Part model, mm, in its own coordinate system. A direction names the side the tool comes from. Round coordinates to 2 decimals unless told otherwise and drop trailing zeros. Loops run counter-clockwise (first coordinate to the right, second up) from the corner with the lowest first, then second, coordinate; pieces in that order, holes last. Notation, with made-up numbers: (13.25, 31.25) -> (19.25, 31.25) arc R18 cw to (19.25, 60.25) -> close; hole circle Ø5 at (8, 1.25). An arc over 180 degrees is marked (long way). Use a Markdown table: item, result. Add a question column.
Item 1: Flat gauge pins, fed straight in: pin 1 (6 mm diameter, centred on y = -8.5, z = -14.5, fed in from +X); pin 2 (5 mm diameter, centred on x = 40.5, y = 12, fed in from -Z); pin 3 (12 mm diameter, centred on y = -21, z = -41.5, fed in from +X). Where does each tip first touch, or does it go through?
Item 2: Probe line 1 (Z direction, x = 0, y = -21); line 2 (Z direction, x = 0, y = -1.25). List the from-to ranges inside material, lowest first. Write a range as [from, to].
Item 3: Cut at C-C, the plane y = -18.5. List the corners of the cut face in (x, z).
Item 4: Cut at A-A, the plane x = 0. List the corners of the cut face in (y, z) (3 decimals).
Item 5: Cut at B-B, the plane z = 0. List the corners of the cut face in (x, y) (3 decimals).
Item 6: Two-plate mould, pull along Z, no slides. Class faces 1 (the face through (-66.746, -25.222, 21.019)), 2 (the face through (-59, -38.1, 38)), 3 (the face through (14.481, -4.171, -65.213)), 4 (the face through (15.86, -25.58, 71.41)): pulls with the +Z half, pulls with the -Z half, needs draft (parallel to the pull), parting line crosses it, or undercut.
Item 7: Which spindle directions (+Z, -Z, +X, -X, +Y, -Y) get a long thin tool onto all of the face, cutting with end or side? Do faces 5 (the face through (-14, 4.123, -45)), 6 (the face through (73.068, 12.522, 56.026)), 7 (the face through (75.587, -6.439, 57.958)). Say none if no direction does.
Autodesk Inventor part; units mm, degrees
ref_plane "YZ Plane" through (0, 0, 0) normal (1, 0, 0) x (0, 1, 0)
ref_plane "XZ Plane" through (0, 0, 0) normal (0, 1, 0) x (-1, 0, 0)
ref_plane "XY Plane" through (0, 0, 0) normal (0, 0, 1) x (1, 0, 0)
sketch "Sketch1" plane through (0, 0, 0) normal (0, 0, 1) x (1, 0, 0)
  line L0 (0, 25.4) -> (-28.702, 25.4) construction
  line L1 (0, 25.4) -> (-95.25, 25.4) construction
  line L2 (-95.25, 25.4) -> (-92.075, 25.4) construction
  line L3 (-92.075, 25.4) -> (-84.455, 21.8467) construction
  line L4 (-92.075, 25.4) -> (-92.075, 22.4389) construction
  line L5 (-92.075, 0) -> (-95.25, 0)
  line L6 (-28.702, 59.0535) -> (-28.702, -92.5226) construction
  arc A0 (-28.9184, -9.8402) -> (-32.3684, -2.4417) centre (-35.052, -8.1967) ccw
  line L7 (-76.2, -186.2977) -> (-28.702, -9.0327)
  line L8 (-92.075, 25.4) -> (-92.075, 0)
  line L9 (-92.075, 25.4) -> (-32.3684, -2.4417)
  line L10 (-28.702, -8.1967) -> (-60.452, -8.1967) construction
  line L11 (-60.452, -127.5253) -> (-54.102, -127.5253) construction
  line L12 (-54.102, -127.5253) -> (-54.102, -103.8268) construction
  line L13 (-54.102, -103.8268) -> (-60.452, -103.8268)
  line L14 (-60.452, 10.654) -> (-60.452, 1.129) construction
  line L15 (-60.452, 10.654) -> (-60.452, 4.1232) construction
  line L16 (-60.452, 4.1232) -> (-46.4468, 4.1232)
  line L17 (-95.25, 0) -> (-95.25, -12.7) construction
  line L18 (-60.452, -12.7) -> (-73.152, -12.7) construction
  line L19 (-95.25, -12.7) -> (-95.25, -25.4) construction
  line L20 (-95.25, -25.4) -> (-95.25, -88.9) construction
  line L21 (-95.25, -88.9) -> (-82.55, -88.9) construction
  line L22 (-82.55, -88.9) -> (-82.55, -25.4) construction
  line L23 (-95.25, -25.4) -> (-82.55, -25.4)
  line L24 (-82.55, -25.4) -> (-82.55, -88.9)
  line L25 (-82.55, -88.9) -> (-95.25, -88.9)
  line L26 (-95.25, -12.7) -> (-73.152, -12.7)
  line L27 (-73.152, -139.3746) -> (-63.627, -139.3746)
  line L28 (-82.55, -88.9) -> (-82.55, -186.2977)
  line L29 (-82.55, -186.2977) -> (-76.2, -186.2977)
  line L30 (-73.152, -12.7) -> (-73.152, -139.3746)
  line L31 (-88.9, -25.4) -> (-88.9, -31.3436)
  line L32 (-88.9, -31.3436) -> (-95.25, -31.3436)
  line L33 (-95.25, 0) -> (-95.25, -25.4)
  line L34 (-95.25, -31.3436) -> (-95.25, -88.9)
  line L35 (-88.9, -160.8977) -> (-88.9, -221.8454)
  line L36 (-28.9184, -9.8402) -> (-85.725, -221.8454)
  line L37 (-85.725, -221.8454) -> (-88.9, -221.8454)
  line L38 (-82.55, -160.8977) -> (-88.9, -160.8977)
  line L39 (-66.802, -38.1) -> (-66.802, 4.1232)
  line L40 (-66.802, 4.1232) -> (-60.452, 4.1232)
  line L41 (-66.802, -38.1) -> (-60.452, -103.8268)
  line L42 (-60.452, 10.654) -> (-60.452, 4.1232) construction
  line L43 (-60.452, -8.1967) -> (-60.452, -12.7) construction
  line L44 (-60.452, -103.8268) -> (-60.452, -127.5253) construction
  line L45 (0, 59.6457) -> (0, -91.9304) construction
  line L46 (-73.152, -38.1) -> (-69.977, -38.1)
  line L47 (-69.977, -38.1) -> (-69.977, -12.7)
  line L48 (-66.802, -12.7) -> (-69.977, -12.7)
  point P0 (0, 0)
  point P1 (-95.25, -256.5049)
  point P2 (-88.7095, 22.4389)
  dimension "d0" = 28.702
  dimension "d1" = 95.25
  dimension "d2" = 3.175
  dimension "d3" = 25
  dimension "d5" = 25.4
  dimension "d6" = 25.4
  dimension "d8" = 12.7
  dimension "d12" = 31.75
  dimension "d13" = 6.35
  dimension "d16" = 12.7
  dimension "d17" = 12.7
  dimension "d18" = 12.7
  dimension "d19" = 63.5
  dimension "d20" = 12.7
  dimension "d22" = 9.525
  dimension "d23" = 6.35
  dimension "d25" = 5.9436
  dimension "d27" = 3.175
  dimension "d28" = 6.35
  dimension "d29" = 25.4
  dimension "d30" = 107.95
  dimension "d31" = 6.35
  dimension "d33" = 20.3552
  dimension "d34" = 15
  dimension "d35" = 3.175
  dimension "d36" = 25.4
revolve "Revolution1" add sketch "Sketch1" angle 360 about axis through (0, 59.6457, 0) along (0, -1, 0) contours L8 L9 L16 L40 L39 L48 L47 L46 L30 L26 L33 L5
properties part number "phenolic_top" material "Phenolic Resin"
A:
| question | item | result |
|---|---|---|
| 1 | pin 1 | stops at x = 94.55 |
| 1 | pin 2 | stops at z = -83.87 |
| 1 | pin 3 | stops at x = 63.96 |
| 2 | line 1 | z = [-73.15, -69.98], [69.98, 73.15] |
| 2 | line 2 | z = [-95.25, -66.8], [66.8, 95.25] |
| 3 | outline | circle Ø146.3 at (0, 0); hole circle Ø139.95 at (0, 0) |
| 4 | outline | (-38.1, -73.152) -> (-12.7, -73.152) -> (-12.7, -95.25) -> (0, -95.25) -> (0, -92.075) -> (25.4, -92.075) -> (4.123, -46.447) -> (4.123, -66.802) -> (-12.7, -66.802) -> (-12.7, -69.977) -> (-38.1, -69.977) -> close; (-38.1, 69.977) -> (-12.7, 69.977) -> (-12.7, 66.802) -> (4.123, 66.802) -> (4.123, 46.447) -> (25.4, 92.075) -> (0, 92.075) -> (0, 95.25) -> (-12.7, 95.25) -> (-12.7, 73.152) -> (-38.1, 73.152) -> close |
| 5 | outline | (-95.25, -12.7) -> (-73.152, -12.7) -> (-73.152, -38.1) -> (-69.977, -38.1) -> (-69.977, -12.7) -> (-66.802, -12.7) -> (-66.802, 4.123) -> (-46.447, 4.123) -> (-92.075, 25.4) -> (-92.075, 0) -> (-95.25, 0) -> close; (46.447, 4.123) -> (66.802, 4.123) -> (66.802, -12.7) -> (69.977, -12.7) -> (69.977, -38.1) -> (73.152, -38.1) -> (73.152, -12.7) -> (95.25, -12.7) -> (95.25, 0) -> (92.075, 0) -> (92.075, 25.4) -> close |
| 6 | face 1 | undercut |
| 6 | face 2 | needs draft |
| 6 | face 3 | undercut |
| 6 | face 4 | parting line crosses it |
| 7 | face 5 | -Y |
| 7 | face 6 | +Y |
| 7 | face 7 | +Y, -Y |
